Could you check a few things on this model? Use its own coordinates, in mm. A direction names the side the tool comes from. Give positions to 0.01 mm unless a question says otherwise; leave off trailing zeros. Loops run counter-clockwise (first coordinate to the right, second up) from the corner with the lowest first, then second, coordinate; pieces in that order, holes last. Notation, with made-up numbers: M 77,53.5 L 132,53.5 A26 ccw 132,86.5 Z; hole C 44,23.25 d2. An arc over 180 degrees is marked long. Use a Markdown table: item, result. Add a question column.
1) If I drill on line 1 along Y through (x, z) = (0, 26) (3 decimals); line 2 along Y through (x, z) = (-0.2, -29); line 3 along Z through (x, y) = (-0.05, -1.5), over which ranges is the centre line in solid material (lowest first)? Write a range as [from, to].
2) Suppose I cut it at C-C on y = -2. List the corners of the cut face in (x, z) for me.
3) Which directions (+Z, -Z, +X, -X, +Y, -Y) give clear straight access to the entire face, cutting with the end or side of a thin tool? Please do faces 4 (the flat face through (0, -6.042, -37)), 5 (the cylindrical face through (0, 0, 55)).
4) We'd pull the mould along Z, two halves only. Please class faces 1 (the flat face through (-1.25, 0, 1)), 2 (the cylindrical face through (0, 0, -55)), 3 (the flat face through (-0.02, -4.56, -24.62)): +Z half, -Z half, draft (parallel to the pull), parting line (faces both ways), or undercut.
5) Suppose I cut it at D-D on y = 8.5. List the corners of the cut face in (x, z) for me.
6) Will these pins go through, and if not, where does the flat tip stop? pin 1 Ø1.2 at (x, y) = (0, -2.5) entering from +Z; pin 2 Ø1 at (x, y) = (-0.5, 3) entering from -Z; pin 3 Ø1 at (x, y) = (0.5, -7.5) entering from -Z.
7) Suppose I cut it at B-B on x = -0.15. Count the separate pieces of the cut face and the enclosed holes in it, and give its area (3 significant figures).
8) Suppose I cut it at A-A on z = -37. List the corners of the cut face in (x, y) for me, and give its area (3 significant figures).
```python
from build123d import *

# Parameters (mm, degrees)
SKETCH1_W               = 110
SKETCH1_H               = 20
BOSS_EXTRUDE1_DEPTH     = 1.25
CUT_EXTRUDE1_DEPTH      = 56.957573214
CUT_EXTRUDE1_DEPTH_BACK = 56.957573214
SKETCH2_R               = 1.1
CUT_EXTRUDE2_DEPTH      = 56.957573214
CUT_EXTRUDE2_DEPTH_BACK = 56.957573214
SKETCH3_R               = 0.675
CUT_EXTRUDE3_DEPTH      = 56.957573214
CUT_EXTRUDE3_DEPTH_BACK = 56.957573214
FILLET2_RADIUS          = 10
FILLET2_LENGTH          = 2.5
FILLET3_RADIUS          = 10
FILLET3_LENGTH          = 2.5


with BuildPart() as part:
    # Sketch1 → Boss-Extrude1 (new, symmetric)
    with BuildSketch(Plane(origin=(0, 0, 0), x_dir=(0, 0, -1), z_dir=(1, 0, 0))):
        Rectangle(SKETCH1_W, SKETCH1_H)
    extrude(amount=BOSS_EXTRUDE1_DEPTH, both=True)

    # Sketch2 → Cut-Extrude1 (cut, two sides: drawn at the far end of the back side and taken through both)
    with BuildSketch(Plane(origin=(1.25, 0, 0), x_dir=(0, 0, -1), z_dir=(1, 0, 0)).offset(-CUT_EXTRUDE1_DEPTH_BACK)):
        with Locations((-35, 0)):
            Circle(SKETCH2_R)
    extrude(amount=CUT_EXTRUDE1_DEPTH + CUT_EXTRUDE1_DEPTH_BACK, mode=Mode.SUBTRACT)

    # Sketch3 → Cut-Extrude2 (cut, two sides: drawn at the far end of the back side and taken through both)
    with BuildSketch(Plane(origin=(1.25, 0, 0), x_dir=(0, 0, -1), z_dir=(1, 0, 0)).offset(-CUT_EXTRUDE2_DEPTH_BACK)):
        with Locations((-50.6, 0)):
            Circle(SKETCH3_R)
        with Locations((-48.4, 0)):
            Circle(SKETCH3_R)
        with Locations((-46.2, 0)):
            Circle(SKETCH3_R)
        with Locations((-44, 0)):
            Circle(SKETCH3_R)
        with Locations((-41.8, 0)):
            Circle(SKETCH3_R)
        with Locations((-39.6, 0)):
            Circle(SKETCH3_R)
        with Locations((-30.4, 0)):
            Circle(SKETCH3_R)
        with Locations((-28.2, 0)):
            Circle(SKETCH3_R)
        with Locations((-26, 0)):
            Circle(SKETCH3_R)
        with Locations((-23.8, 0)):
            Circle(SKETCH3_R)
        with Locations((-21.6, 0)):
            Circle(SKETCH3_R)
        with Locations((-19.4, 0)):
            Circle(SKETCH3_R)
    extrude(amount=CUT_EXTRUDE2_DEPTH + CUT_EXTRUDE2_DEPTH_BACK, mode=Mode.SUBTRACT)

    # Sketch4 → Cut-Extrude3 (cut, two sides: drawn at the far end of the back side and taken through both)
    with BuildSketch(Plane(origin=(1.25, 0, 0), x_dir=(0, 0, -1), z_dir=(1, 0, 0)).offset(-CUT_EXTRUDE3_DEPTH_BACK)):
        Polygon((25.569688234, -6.041537935), (48, -6.041537935), (48, 6.041537935), (25.569688234, 6.041537935), (23.701172911, 3.12608256), (23.701172911, -3.12608256), align=None)
    extrude(amount=CUT_EXTRUDE3_DEPTH + CUT_EXTRUDE3_DEPTH_BACK, mode=Mode.SUBTRACT)

    # Fillet2: full round fillet: the end face becomes a half cylinder, R = half its width
    fillet2_face = Plane((0, 0, -55), x_dir=(-1, 0, 0), z_dir=(0, 0, -1))  # on the end face: x along it, z out of the body
    fillet2_slab = fillet2_face.offset(-FILLET2_RADIUS / 2) * Box(FILLET2_LENGTH, 2 * FILLET2_RADIUS, FILLET2_RADIUS, mode=Mode.PRIVATE)  # the body's end, R deep
    fillet2_round = Plane((0, 0, -45), x_dir=(0, 0, -1), z_dir=(-1, 0, 0)) * Cylinder(FILLET2_RADIUS, FILLET2_LENGTH, mode=Mode.PRIVATE)  # its axis R under the face
    add(fillet2_slab - fillet2_round, mode=Mode.SUBTRACT)

    # Fillet3: full round fillet: the end face becomes a half cylinder, R = half its width
    fillet3_face = Plane((0, 0, 55), x_dir=(1, 0, 0), z_dir=(0, 0, 1))  # on the end face: x along it, z out of the body
    fillet3_slab = fillet3_face.offset(-FILLET3_RADIUS / 2) * Box(FILLET3_LENGTH, 2 * FILLET3_RADIUS, FILLET3_RADIUS, mode=Mode.PRIVATE)  # the body's end, R deep
    fillet3_round = Plane((0, 0, 45), x_dir=(0, 0, 1), z_dir=(1, 0, 0)) * Cylinder(FILLET3_RADIUS, FILLET3_LENGTH, mode=Mode.PRIVATE)  # its axis R under the face
    add(fillet3_slab - fillet3_round, mode=Mode.SUBTRACT)


solid = part.part
```
Answer block:
| question | item | result |
|---|---|---|
| 1 | line 1 | y = [-10, -0.675], [0.675, 10] |
| 1 | line 2 | y = [-10, -6.04], [6.04, 10] |
| 1 | line 3 | z = [-54.89, -48], [-23.7, 54.89] |
| 2 | outline | M -1.25,-54.8 L 1.25,-54.8 L 1.25,-48 L -1.25,-48 Z; M -1.25,-23.7 L 1.25,-23.7 L 1.25,54.8 L -1.25,54.8 Z |
| 3 | face 4 | +X, -X |
| 3 | face 5 | +Z, +X, -X |
| 4 | face 1 | draft |
| 4 | face 2 | -Z half |
| 4 | face 3 | undercut |
| 5 | outline | M -1.25,-50.27 L 1.25,-50.27 L 1.25,50.27 L -1.25,50.27 Z |
| 6 | pin 1 | stops at z = 54.82 |
| 6 | pin 2 | stops at z = -54.68 |
| 6 | pin 3 | stops at z = -52.14 |
| 7 | separate pieces | 1 |
| 7 | enclosed holes | 14 |
| 7 | area | 1,810 mm^2 |
| 8 | outline | M -1.25,-10 L 1.25,-10 L 1.25,-6.04 L -1.25,-6.04 Z; M -1.25,6.04 L 1.25,6.04 L 1.25,10 L -1.25,10 Z |
| 8 | area | 19.8 mm^2 |
